from build123d import *

# Parameters (mm, degrees)
F0_R          = 7
F0_R_2        = 5.5
F1_DEPTH      = 5
F1_DEPTH_BACK = 5
F2_R          = 0.5
F3_DEPTH      = 4
F3_DEPTH_BACK = 4


with BuildPart() as f1:
    # F0 (on Top) → F1 (new body, two sides)
    with BuildSketch(Plane.XY) as f1_sk:
        Circle(F0_R)
        Circle(F0_R_2, mode=Mode.SUBTRACT)
    extrude(amount=F1_DEPTH)
    extrude(f1_sk.sketch, amount=-F1_DEPTH_BACK)

    # F2 (on Top) → F3 (join, two sides)
    with BuildSketch(Plane.XY) as f3_sk:
        with Locations((0, 5.5)):
            Circle(F2_R)
        with Locations((-1.699593, 5.230811)):
            Circle(F2_R)
        with Locations((-3.232819, 4.449593)):
            Circle(F2_R)
        with Locations((-4.449593, 3.232819)):
            Circle(F2_R)
        with Locations((-5.230811, 1.699593)):
            Circle(F2_R)
        with Locations((-5.5, 0)):
            Circle(F2_R)
        with Locations((-5.230811, -1.699593)):
            Circle(F2_R)
        with Locations((-4.449593, -3.232819)):
            Circle(F2_R)
        with Locations((-3.232819, -4.449593)):
            Circle(F2_R)
        with Locations((-1.699593, -5.230811)):
            Circle(F2_R)
        with Locations((0, -5.5)):
            Circle(F2_R)
        with Locations((1.699593, -5.230811)):
            Circle(F2_R)
        with Locations((3.232819, -4.449593)):
            Circle(F2_R)
        with Locations((4.449593, -3.232819)):
            Circle(F2_R)
        with Locations((5.230811, -1.699593)):
            Circle(F2_R)
        with Locations((5.5, 0)):
            Circle(F2_R)
        with Locations((5.230811, 1.699593)):
            Circle(F2_R)
        with Locations((4.449593, 3.232819)):
            Circle(F2_R)
        with Locations((3.232819, 4.449593)):
            Circle(F2_R)
        with Locations((1.699593, 5.230811)):
            Circle(F2_R)
    extrude(amount=F3_DEPTH)
    extrude(f3_sk.sketch, amount=-F3_DEPTH_BACK)


solid = f1.part
Geometry: final body of the model. Coordinates: model frame, mm. Give positions to 0.01 mm unless a question says otherwise; leave off trailing zeros. Loops run counter-clockwise (first coordinate to the right, second up) from the corner with the lowest first, then second, coordinate; pieces in that order, holes last. Notation, with made-up numbers: (72.25, 54) - (100.25, 54) arc R32 cw to (100.25, 85) - close; hole circle Ø10 at (39, 30). An arc over 180 degrees is marked (long way). Answer as CSV lines item,"result". Start each with the question number.
1. Ray query, L1, parallel to Y at x = -5.25, z = 2.75; L2, parallel to X at y = -3.25, z = 4.75; L3, parallel to X at y = 2.75, z = -4.5. Return the intervals inside material, ascending.
2. Section B-B, the plane y = -4.5. Return loops of the section in (x, z).
3. Section D-D, the plane y = 0.75. Return loops of the section in (x, z), plus the area to 3 significant figures.
4. Pin query (flat end, axial travel): P1, Ø2, axis at x = 3.5, z = 3.5, coming from the -Y side; P2, Ø3, axis at x = -4.5, z = 2.5, coming from the -Y side; P3, Ø2, axis at y = 3.5, z = 0, coming from the +X side; P4, Ø5, axis at y = -0.5, z = 0, coming from the +X side. Return the tip coordinate at first contact, or that it passes through.
5. Section C-C, the plane z = -4.25. Return loops of the section in (x, y).
6. Section A-A, the plane x = 0. Return loops of the section in (y, z).
7. Draft query along X for faces 1 (the face through (4.76, -1.53, 0.06)), 2 (the face through (-4, -4, -5)). Return one class per face: released by +X, released by -X, zero draft, split by the parting line, or undercut.
Answers:
1,L1,"y = -4.63 to -1.2, -0.43 to 0.43, 1.2 to 4.63"
1,L2,"x = -6.2 to -4.44, 4.44 to 6.2"
1,L3,"x = -6.44 to -4.76, 4.76 to 6.44"
2,outline,"(-5.36, -5) - (-3.16, -5) - (-3.16, -4) - (-2.74, -4) - (-2.74, 4) - (-3.16, 4) - (-3.16, 5) - (-5.36, 5) - close; (2.74, -4) - (3.16, -4) - (3.16, -5) - (5.36, -5) - (5.36, 5) - (3.16, 5) - (3.16, 4) - (2.74, 4) - close"
3,outline,"(-6.96, -5) - (-5.45, -5) - (-5.45, 5) - (-6.96, 5) - close; (5.45, -5) - (6.96, -5) - (6.96, 5) - (5.45, 5) - close"
3,area,"30.2 mm2"
4,P1,"stops at y = -6.54"
4,P2,"stops at y = -6.32"
4,P3,"stops at x = 6.54"
4,P4,"stops at x = 7"
5,outline,"circle Ø14 at (0, 0); hole circle Ø11 at (0, 0)"
6,outline,"(-7, -5) - (-5.5, -5) - (-5.5, -4) - (-5, -4) - (-5, 4) - (-5.5, 4) - (-5.5, 5) - (-7, 5) - close; (5, -4) - (5.5, -4) - (5.5, -5) - (7, -5) - (7, 5) - (5.5, 5) - (5.5, 4) - (5, 4) - close"
7,face 1,"undercut"
7,face 2,"zero draft"
